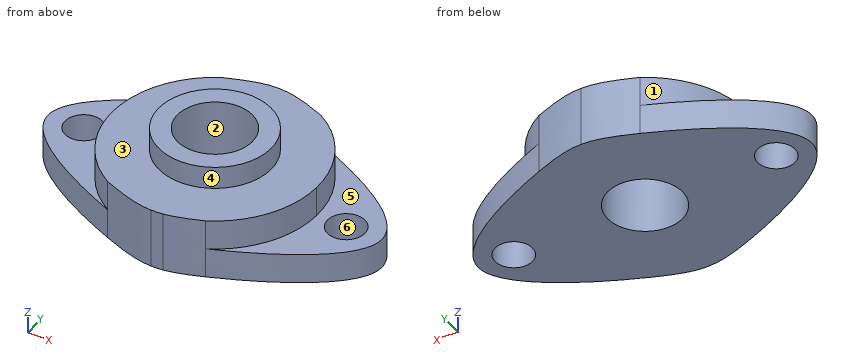
```python
from build123d import *

# Parameters (mm, degrees)
F0_R     = 5
F1_DEPTH = 8
F0_R_2   = 15
F2_DEPTH = 16
F0_R_3   = 10
F3_DEPTH = 22


with BuildPart() as f1:
    # F0 (on Top) → F1 (new body)
    with BuildSketch(Plane.XY):
        with BuildLine():
            ThreePointArc((-14.128437921, -23.593160914), (-27.4985146505, 0.2858181561), (-13.6349863045, 23.8817325267))
            add(Edge.make_bspline(
                [(-13.6349863045, 23.8817325267), (-24.80887432, 19.3175732433), (-64.9074286316, -0.0208843712), (-25.3732238209, -18.9980920778), (-14.128437921, -23.593160914)],
                knots=[0.0936300618, 0.0936300618, 0.0936300618, 0.0936300618, 0.2501498665, 0.4055392908, 0.4055392908, 0.4055392908, 0.4055392908], degree=3))
        make_face()
        with Locations((-35.5, 0)):
            Circle(F0_R, mode=Mode.SUBTRACT)
    extrude(amount=F1_DEPTH)



with BuildPart() as f1b:
    # F0 (on Top) → F1, piece 2 (new body)
    with BuildSketch(Plane.XY):
        with BuildLine():
            add(Edge.make_bspline(
                [(12.8034054524, -24.3376828976), (23.9154797228, -19.8963977435), (65.6301130949, 0.0418102706), (24.8166936559, 19.3644997944), (13.6114848151, 23.8951350933)],
                knots=[0.5915126143, 0.5915126143, 0.5915126143, 0.5915126143, 0.7498837302, 0.9064567635, 0.9064567635, 0.9064567635, 0.9064567635], degree=3))
            ThreePointArc((13.6114848151, 23.8951350933), (23.7756790904, 13.8190840432), (27.5, 0))
            ThreePointArc((27.5, 0), (23.5408543806, -14.2154203255), (12.8034054524, -24.3376828976))
        make_face()
        with Locations((35.5, 0)):
            Circle(F0_R, mode=Mode.SUBTRACT)
    extrude(amount=F1_DEPTH)


with BuildPart() as f1_1:
    add(f1.part)

    add(f1b.part)  # F2 merges F1b
    # F0 (on Top) → F2 (join)
    with BuildSketch(Plane.XY):
        with BuildLine():
            add(Edge.make_bspline(
                [(13.6114848151, 23.8951350933), (6.9170274268, 26.6019248892), (3.4653354317, 27.4970657947), (0, 27.5)],
                knots=[0.9064567635, 0.9064567635, 0.9064567635, 0.9064567635, 1, 1, 1, 1], degree=3))
            add(Edge.make_bspline(
                [(0, 27.5), (-3.4685519028, 27.5029369288), (-6.9507725812, 26.6120101235), (-13.6349863045, 23.8817325267)],
                knots=[0, 0, 0, 0, 0.0936300618, 0.0936300618, 0.0936300618, 0.0936300618], degree=3))
            ThreePointArc((-13.6349863045, 23.8817325267), (-27.4985146505, 0.2858181561), (-14.128437921, -23.593160914))
            add(Edge.make_bspline(
                [(-14.128437921, -23.593160914), (-7.2216478267, -26.4155513269), (-3.503029764, -27.4047401273), (0, -27.5)],
                knots=[0.4055392908, 0.4055392908, 0.4055392908, 0.4055392908, 0.5009828275, 0.5009828275, 0.5009828275, 0.5009828275], degree=3))
            ThreePointArc((0, -27.5), (1.5905265483, -27.453965566), (3.1757280792, -27.3160163854))
            add(Edge.make_bspline(
                [(3.1757280792, -27.3160163854), (5.6032444341, -26.9627476234), (8.4443384991, -26.079919214), (12.8034054524, -24.3376828976)],
                knots=[0.5293864729, 0.5293864729, 0.5293864729, 0.5293864729, 0.5915126143, 0.5915126143, 0.5915126143, 0.5915126143], degree=3))
            ThreePointArc((12.8034054524, -24.3376828976), (23.5408543806, -14.2154203255), (27.5, 0))
            ThreePointArc((27.5, 0), (23.7756790904, 13.8190840432), (13.6114848151, 23.8951350933))
        make_face()
        Circle(F0_R_2, mode=Mode.SUBTRACT)
    extrude(amount=F2_DEPTH)

    # F0 (on Top) → F3 (join)
    with BuildSketch(Plane.XY):
        Circle(F0_R_2)
        Circle(F0_R_3, mode=Mode.SUBTRACT)
    extrude(amount=F3_DEPTH)


solid = f1_1.part
```
CAD build for the part. Positions are in the model's coordinates, mm. Face numbers are marked on the shaded views. A direction names the side the tool comes from. Round coordinates to 2 decimals unless told otherwise and drop trailing zeros. Order: outer loops, then holes, each group sorted by start corner. A loop starts at its lowest first (then second) coordinate and runs counter-clockwise, first axis right, second up.
Q1. Drop flat-ended pins along their axis: pin 1 (2 mm diameter, centred on x = 22, z = 13.5, fed in from +Y); pin 2 (1 mm diameter, centred on y = 3.5, z = 17, fed in from +X); pin 3 (1.5 mm diameter, centred on x = 21, z = 14.5, fed in from +Y). Give the stop position or say it passes through.
Q2. Which spindle directions (+Z, -Z, +X, -X, +Y, -Y) get a long thin tool onto all of the face, cutting with end or side? Do the marked faces 1, 2 and 3. Say none if no direction does.
Q3. Slice it at B-B (z = 5.25). State how many separate pieces and enclosed holes the cut face has, and give its area (3 significant figures).
Q4. Two-plate mould, pull along X, no slides. Class the marked faces 4, 5 and 6: pulls with the +X half, pulls with the -X half, needs draft (parallel to the pull), parting line crosses it, or undercut.
Q5. Slice it at A-A (z = 19). Write the cut outline in (x, y), and give its area (3 significant figures).
Q6. Wall check: L1, parallel to Y at x = 0, z = 10; L2, parallel to Z at x = 23.5, y = 6; L3, parallel to Y at x = 35.5, z = 2. Give the ranges that are in metal, low to high.
Results below:
1. pin 1: stops at y = 17.76
1. pin 2: stops at x = 14.7
1. pin 3: stops at y = 18.61
2. face 1: +Z, -X
2. face 2: +Z, -Z
2. face 3: +Z
3. separate pieces: 1
3. enclosed holes: 3
3. area: 2,900 mm2
4. face 4: parting line crosses it
4. face 5: needs draft
4. face 6: undercut
5. outline: circle Ø30 at (0, 0); hole circle Ø20 at (0, 0)
5. area: 393 mm2
6. L1: y = -27.5 to -10, 10 to 27.5
6. L2: z = 0 to 16
6. L3: y = -12.53 to -5, 5 to 12.59
